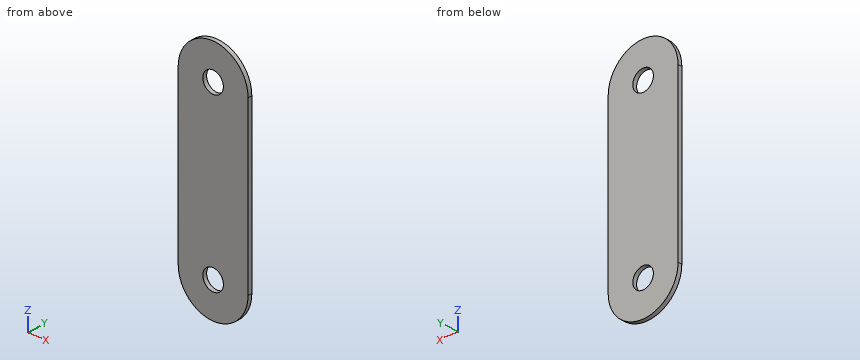
Solid Edge part; units mm, degrees
sketch "Sketch1" plane through (0, 0, 0) normal (0, -1, 0) x (1, 0, 0)
  line L0 (8.5, 0) -> (8.5, 40.64)
  line L1 (-8.5, 40.64) -> (-8.5, 0)
  arc A0 (-8.5, 40.64) -> (8.5, 40.64) centre (0, 40.64) cw
  arc A1 (8.5, 0) -> (-8.5, 0) centre (0, 0) cw
  circle A2 centre (0, 40.64) radius 2.5
  circle A3 centre (0, 0) radius 2.5
extrude "Protrusion1" add sketch "Sketch1" against normal blind 1
Check sheet for the modelled part. Datum: model origin and axes. Units: mm. Give positions to 0.01 mm unless a question says otherwise; leave off trailing zeros. Loops run counter-clockwise (first coordinate to the right, second up) from the corner with the lowest first, then second, coordinate; pieces in that order, holes last. Notation, with made-up numbers: M 29,7 L 58,7 A25 ccw 58,19 Z; hole C 17,-36 d8. An arc over 180 degrees is marked long. Answer as a JSON object with one key per item and string values. Group by question number.
Q1. Cross-section at D-D on z = 42.5. Record the cut outline in (x, y).
Q2. Cross-section at C-C on y = 0.6. Record the cut outline in (x, z).
Q3. Cross-section at B-B on z = -1. Record the cut outline in (x, y), then the cut area to 3 significant figures.
Q4. Cross-section at A-A on x = 0. Record the cut outline in (y, z).
Q5. Material ranges on line 1 along Z through (x, y) = (0, 0.35); line 2 along Z through (x, y) = (-1, 0.7); line 3 along X through (y, z) = (0.75, -1.5), recorded low to high. Write a range as [from, to].
Evaluation:
{
 "1": {"outline": "M -8.29,0 L -1.67,0 L -1.67,1 L -8.29,1 Z; M 1.67,0 L 8.29,0 L 8.29,1 L 1.67,1 Z"},
 "2": {"outline": "M -8.5,0 A8.5 ccw 8.5,0 L 8.5,40.64 A8.5 ccw -8.5,40.64 Z; hole C 0,0 d5; hole C 0,40.64 d5"},
 "3": {"outline": "M -8.44,0 L -2.29,0 L -2.29,1 L -8.44,1 Z; M 2.29,0 L 8.44,0 L 8.44,1 L 2.29,1 Z", "area": "12.3 mm2"},
 "4": {"outline": "M 0,-8.5 L 1,-8.5 L 1,-2.5 L 0,-2.5 Z; M 0,2.5 L 1,2.5 L 1,38.14 L 0,38.14 Z; M 0,43.14 L 1,43.14 L 1,49.14 L 0,49.14 Z"},
 "5": {"line 1": "z = [-8.5, -2.5], [2.5, 38.14], [43.14, 49.14]", "line 2": "z = [-8.44, -2.29], [2.29, 38.35], [42.93, 49.08]", "line 3": "x = [-8.37, -2], [2, 8.37]"}
}
